```python
from build123d import *

# Parameters (mm, degrees)
SKETCH1_W           = 114.3
SKETCH1_H           = 203.2
BOSS_EXTRUDE1_DEPTH = 88.9
CUT_EXTRUDE1_DEPTH  = 115.3
FILLET1_R           = 25.24
FILLET2_R           = 15.08
CUT_EXTRUDE2_DEPTH  = 115.3
LPATTERN1_COUNT     = 2
LPATTERN1_PITCH     = 101.6
SHELL5_T            = -1.27
SKETCH9_R           = 3
BOSS_EXTRUDE2_DEPTH = 8.89


with BuildPart() as part:
    # Sketch1 → Boss-Extrude1 (new body)
    with BuildSketch(Plane(origin=(0, 0, 0), x_dir=(0, 0, -1), z_dir=(1, 0, 0))):
        with Locations((57.15, -101.6)):
            Rectangle(SKETCH1_W, SKETCH1_H)
    extrude(amount=-BOSS_EXTRUDE1_DEPTH)

    # Sketch4 → Cut-Extrude1 (cut, through all)
    with BuildSketch(Plane(origin=(0, 0, -114.3), x_dir=(-1, 0, 0), z_dir=(0, 0, -1))):
        Polygon((88.9, 0), (63.5, 0), (88.9, -101.6), align=None)
        Polygon((88.9, -203.2), (88.9, -101.6), (63.5, -203.2), align=None)
    extrude(amount=-CUT_EXTRUDE1_DEPTH, mode=Mode.SUBTRACT)

    # Fillet1
    fillet1_edges = [part.edges().sort_by_distance(p)[0] for p in [
        (-88.9, -101.6, -57.15),
    ]]
    fillet(fillet1_edges, radius=FILLET1_R)

    # Fillet2
    fillet2_edges = [part.edges().sort_by_distance(p)[0] for p in [
        (-63.5, 0, -57.15),
        (-63.5, -203.2, -57.15),
    ]]
    fillet(fillet2_edges, radius=FILLET2_R)

    # Sketch5 → Cut-Extrude2 (cut, through all)
    with BuildSketch(Plane.XY):
        with BuildLine():
            Line((-12.7, -187.325), (0, -187.325))
            Line((0, -187.325), (0, -117.475))
            Line((0, -117.475), (-12.7, -117.475))
            ThreePointArc((-12.7, -117.475), (-47.625, -152.4), (-12.7, -187.325))
        make_face()
    cut_extrude2 = extrude(amount=-CUT_EXTRUDE2_DEPTH, mode=Mode.SUBTRACT)

    # LPattern1: Cut-Extrude2 ×2
    with Locations(*[(0, i * LPATTERN1_PITCH, 0) for i in range(1, LPATTERN1_COUNT)]):
        add(cut_extrude2, mode=Mode.SUBTRACT)

    # Shell5
    shell5_openings = [part.faces().sort_by_distance(p)[0] for p in [
        (0, -195.2625, -57.15),
        (0, -101.6, -57.15),
        (-30.1625, -152.4, -57.15),
        (-6.35, -117.475, -57.15),
        (-6.35, -187.325, -57.15),
        (0, -7.9375, -57.15),
        (-30.1625, -50.8, -57.15),
        (-6.35, -15.875, -57.15),
        (-6.35, -85.725, -57.15),
    ]]
    offset(amount=SHELL5_T, openings=shell5_openings, kind=Kind.INTERSECTION)

    # Sketch9 → Boss-Extrude2 (add)
    with BuildSketch(Plane.XY.offset(-113.03)):
        with Locations((-12.7, -101.6)):
            Circle(SKETCH9_R)
    boss_extrude2 = extrude(amount=BOSS_EXTRUDE2_DEPTH)

    # Mirror1: Boss-Extrude2 across plane
    add(boss_extrude2.mirror(Plane.XY.offset(-57.15)))


solid = part.part
```
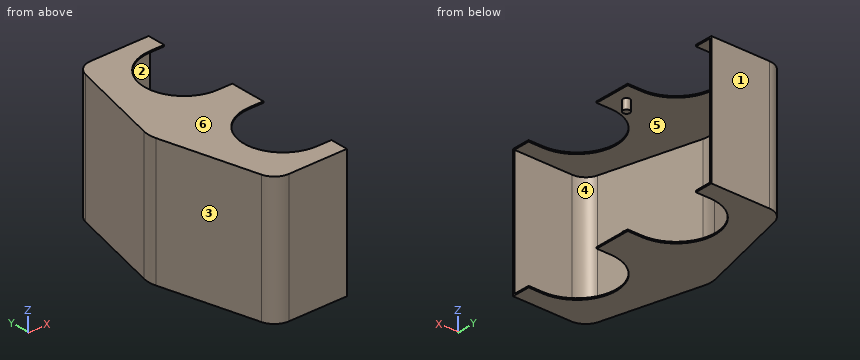
Can you work these out from the model? Positions are in its coordinate system, mm. Face numbers are marked on the shaded views. A direction names the side the tool comes from. Coordinates: 2 decimals unless noted, no trailing zeros. Loops run counter-clockwise (first coordinate to the right, second up) from the corner with the lowest first, then second, coordinate; pieces in that order, holes last.
Item 1: Which directions (+Z, -Z, +X, -X, +Y, -Y) give clear straight access to the entire face, cutting with the end or side of a thin tool? Please do the marked faces 4, 5 and 6.
Answers below:
face 4: +X
face 5: none
face 6: +Z, +X, -X, +Y, -Y
Item 2: Please list where these lines run through material, in increasing order: L1, parallel to Y at x = -14, z = -13.5; L2, parallel to Z at x = -51, y = -37.5; L3, parallel to Y at x = -62, z = -58.5.
Answers below:
L1: y = -203.2 to -201.93, -1.27 to 0
L2: z = -114.3 to -113.03, -1.27 to 0
L3: y = -199.16 to -197.35, -5.85 to -4.04
Item 3: Suppose I cut it at A-A (x = -7). Please give me the cut outline in (y, z) (3 decimals).
Answers below:
outline: (-203.2, -114.3) - (-187.325, -114.3) - (-187.325, -113.03) - (-201.93, -113.03) - (-201.93, -1.27) - (-187.325, -1.27) - (-187.325, 0) - (-203.2, 0) - close; (-117.475, -114.3) - (-85.725, -114.3) - (-85.725, -113.03) - (-117.475, -113.03) - close; (-117.475, -1.27) - (-85.725, -1.27) - (-85.725, 0) - (-117.475, 0) - close; (-15.875, -114.3) - (0, -114.3) - (0, 0) - (-15.875, 0) - (-15.875, -1.27) - (-1.27, -1.27) - (-1.27, -113.03) - (-15.875, -113.03) - close
Item 4: Suppose I cut it at D-D (x = -55.5). Please give me the cut outline in (y, z).
Answers below:
outline: (-202.72, -114.3) - (-0.48, -114.3) - (-0.48, 0) - (-202.72, 0) - close; hole (-201.4, -113.03) - (-1.8, -113.03) - (-1.8, -1.27) - (-201.4, -1.27) - close
Item 5: If we mould it in two halves opening along Y, with no side actions, what happens to the marked faces 1, 2 and 3? For each: released by +Y, released by -Y, zero draft, split by the parting line, or undercut.
Answers below:
face 1: released by +Y
face 2: undercut
face 3: released by -Y
Item 6: Suppose I cut it at B-B (y = -101.6). Please give me the cut outline in (x, z), then the cut area to 3 significant figures.
Answers below:
outline: (-88.12, -114.3) - (0, -114.3) - (0, -113.03) - (-9.7, -113.03) - (-9.7, -104.14) - (-15.7, -104.14) - (-15.7, -113.03) - (-86.85, -113.03) - (-86.85, -1.27) - (-15.7, -1.27) - (-15.7, -10.16) - (-9.7, -10.16) - (-9.7, -1.27) - (0, -1.27) - (0, 0) - (-88.12, 0) - close
area: 472 mm2
Item 7: I'm going to push flat-ended pins straight in: pin 1 (1 mm diameter, centred on y = -117, z = -76.5, fed in from +X); pin 2 (5 mm diameter, centred on y = -170, z = -69.5, fed in from +X); pin 3 (1 mm diameter, centred on x = -54.5, z = -84.5, fed in from +Y). Where does each tip first touch, or does it pass through?
Answers below:
pin 1: stops at x = -83.62
pin 2: stops at x = -69.87
pin 3: stops at y = -0.17
Item 8: Suppose I cut it at C-C (z = -14). Please give me the cut outline in (x, y), then the cut area to 3 significant figures.
Answers below:
outline: (-87.37, -107.72) - (-66.36, -191.78) arc R15.08 ccw to (-51.73, -203.2) - (0, -203.2) - (0, -201.93) - (-51.73, -201.93) arc R13.81 cw to (-65.12, -191.47) - (-86.14, -107.41) arc R23.97 cw to (-86.14, -95.79) - (-65.12, -11.73) arc R13.81 cw to (-51.73, -1.27) - (0, -1.27) - (0, 0) - (-51.73, 0) arc R15.08 ccw to (-66.36, -11.42) - (-87.37, -95.48) arc R25.24 ccw to start
area: 415 mm2
